from build123d import *

# Parameters (mm, degrees)
F0_R     = 37.2630205799
F1_DEPTH = 106.4
F3_DEPTH = 86.5
F5_R     = 25.2537141006
F6_DEPTH = 102.8


# Not quite as in the source:
# - a feature names something its author has since deleted; it is built from what else it names


with BuildPart() as f1:
    # F0 (on Top) → F1 (new body)
    with BuildSketch(Plane.XY):
        Circle(F0_R)
    extrude(amount=F1_DEPTH)

    # F2 (on face) → F3 (join)
    with BuildSketch(Plane.XY.offset(106.4)):
        Polygon((4.5720788687, -32.5187220476), (30.4480788261, -12.2998245754), (25.8759999575, 20.2188974722), (-4.5720788687, 32.5187220476), (-30.4480788261, 12.2998245754), (-25.8759999575, -20.2188974722), align=None)
    extrude(amount=-F3_DEPTH)

    # F5 (on face) → F6 (cut)
    with BuildSketch(Plane.XY.offset(106.4)):
        Circle(F5_R)
    extrude(amount=-F6_DEPTH, mode=Mode.SUBTRACT)


solid = f1.part
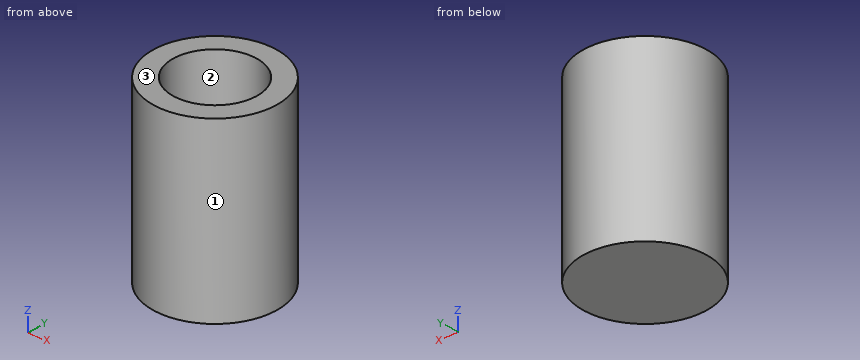
Work out the finished part from the listing and answer in its coordinate system (mm). Face numbers are marked on the shaded views. Round coordinates to 2 decimals unless told otherwise and drop trailing zeros. Loops run counter-clockwise (first coordinate to the right, second up) from the corner with the lowest first, then second, coordinate; pieces in that order, holes last. Notation, with made-up numbers: (-39, 22.5) - (14, 22.5) arc R8 ccw to (14, 35.5) - close; hole circle Ø2 at (14, 39.25). An arc over 180 degrees is marked (long way). Use one line per item in the form item = value. Start each with the question number.
(1) Find section D-D on y = -27.5. Determine the outline of the cut face in (x, z), and give its area (3 significant figures).
(2) Find section C-C on z = 13. Determine the outline of the cut face in (x, y), and give its area (3 significant figures).
(3) Flat-ended cylindrical pins translate along their axes: P1, Ø12, axis at x = -27.5, z = 45, coming from the +Y side; P2, Ø6, axis at x = -4, z = 66.5, coming from the +Y side; P3, Ø4, axis at x = 5.5, z = 59.5, coming from the -Y side. Find the tip coordinate at first contact, or state that the pin passes through.
(4) Determine the mould class of the marked faces 1, 2 and 3 for opening direction X: +X half, -X half, draft (parallel to the pull), parting line (faces both ways), or undercut.
(5) Find section A-A on x = 0. Determine the outline of the cut face in (y, z), and give its area (3 significant figures).
(6) Consider line 1 (Y direction, x = 0, z = 37); line 2 (X direction, y = -16, z = 33). Determine where each line is inside the solid, lowest interval first.
Answer list:
q1.outline = (-25.15, 0) - (25.15, 0) - (25.15, 106.4) - (-25.15, 106.4) - close
q1.area = 5,350 mm^2
q2.outline = circle Ø74.53 at (0, 0); hole circle Ø50.51 at (0, 0)
q2.area = 2,360 mm^2
q3.P1 = 30.43
q3.P2 = 37.25
q3.P3 = -37.1
q4.face_1 = parting line
q4.face_2 = undercut
q4.face_3 = draft
q5.outline = (-37.26, 0) - (37.26, 0) - (37.26, 106.4) - (25.25, 106.4) - (25.25, 3.6) - (-25.25, 3.6) - (-25.25, 106.4) - (-37.26, 106.4) - close
q5.area = 2,740 mm^2
q6.line_1 = -37.26 to -25.25, 25.25 to 37.26
q6.line_2 = -33.65 to -19.54, 19.54 to 33.65
